The listing builds one solid part. Answer for the finished solid, in the listing's coordinates (mm). Coordinates: 2 decimals unless noted, no trailing zeros. Loops run counter-clockwise (first coordinate to the right, second up) from the corner with the lowest first, then second, coordinate; pieces in that order, holes last. Notation, with made-up numbers: (28.5, 69.5) - (47.5, 69.5) arc R23 ccw to (47.5, 89.5) - close; hole circle Ø5 at (85.5, 40.25). An arc over 180 degrees is marked (long way). Return JSON: item names as keys, results as strings. Group by question number.
1. Section A-A (x = 0.65) is taken. Write down the section's boundary in (y, z), and give its area (3 significant figures).
2. Section B-B (x = -0.2) is taken. Write down the section's boundary in (y, z).
3. This flat-tipped pin is pushed along its axis until it touches: P1, Ø1, axis at x = 0.5, z = -3, coming from the -Y side. Where does it stop, or does it pass through?
4. Find the intervals of material crossed by line 1 along Y through (x, z) = (-1.35, 0); line 2 along Y through (x, z) = (0.95, 0); line 3 along Z through (x, y) = (-1.15, 0), in increasing order.
```python
from build123d import *

# Parameters (mm, degrees)
CHAMFER1_SIZE = 0.08


with BuildPart() as part:
    # Sketch1 → Revolve1 (revolve)
    with BuildSketch(Plane.XY):
        with BuildLine():
            Line((-1.1, -3.9), (-0.512347538, -3.9))
            ThreePointArc((-0.512347538, -3.9), (0, -4.15), (0.512347538, -3.9))
            Line((0.512347538, -3.9), (1.1, -3.9))
            Line((1.1, -3.9), (1.1, -4.1))
            Line((1.1, -4.1), (1.3, -4.1))
            Line((1.3, -4.1), (1.3, -4))
            Line((1.3, -4), (1.5, -4))
            Line((1.5, -4), (1.5, -4.5))
            Line((1.5, -4.5), (-1.5, -4.5))
            Line((-1.5, -4.5), (-1.5, -4))
            Line((-1.5, -4), (-1.3, -4))
            Line((-1.3, -4), (-1.3, -4.1))
            Line((-1.3, -4.1), (-1.1, -4.1))
            Line((-1.1, -4.1), (-1.1, -3.9))
        make_face()
    revolve(axis=Axis((-6.429017492, 0, 0), (1, 0, 0)))

    # Chamfer1
    chamfer1_edges = [part.edges().sort_by_distance(p)[0] for p in [
        (1.5, 4.5, 0),
        (-1.5, 4.5, 0),
        (-1.5, 4, 0),
        (1.5, 4, 0),
    ]]
    chamfer(chamfer1_edges, length=CHAMFER1_SIZE)


solid = part.part
```
The answers:
{
 "1": {"outline": "circle Ø9 at (0, 0); hole circle Ø7.8 at (0, 0)", "area": "15.8 mm2"},
 "2": {"outline": "circle Ø9 at (0, 0); hole circle Ø8.24 at (0, 0)"},
 "3": {"P1": "stops at y = -3.74"},
 "4": {"line 1": "y = -4.5 to -4, 4 to 4.5", "line 2": "y = -4.5 to -3.9, 3.9 to 4.5", "line 3": "z = -4.5 to -4.1, 4.1 to 4.5"}
}
